from build123d import *

# Parameters (mm, degrees)
SKETCH1_R           = 2.65
BOSS_EXTRUDE1_DEPTH = 5
BOSS_EXTRUDE2_DEPTH = 10
SKETCH3_R           = 1.4
CUT_EXTRUDE1_DEPTH  = 16


with BuildPart() as part:
    # Sketch1 → Boss-Extrude1 (new body)
    with BuildSketch(Plane.XY):
        with BuildLine():
            Line((5, 28), (-5, 28))
            ThreePointArc((-5, 28), (-23.605754448, 19.060621125), (-28.253479924, -1.05119732))
            ThreePointArc((-28.253479924, -1.05119732), (-23.041182278, -4.770781049), (-18.77, 0))
            ThreePointArc((-18.77, 0), (0, 7.222918877), (18.77, 0))
            ThreePointArc((18.77, 0), (23.041182278, -4.770781049), (28.253479924, -1.05119732))
            ThreePointArc((28.253479924, -1.05119732), (23.605754448, 19.060621125), (5, 28))
        make_face()
        with Locations((-23.57, 0)):
            Circle(SKETCH1_R, mode=Mode.SUBTRACT)
        with Locations((23.57, 0)):
            Circle(SKETCH1_R, mode=Mode.SUBTRACT)
    extrude(amount=BOSS_EXTRUDE1_DEPTH)

    # Sketch2 → Boss-Extrude2 (add)
    with BuildSketch(Plane(origin=(0, 0, 0), x_dir=(-1, 0, 0), z_dir=(0, 0, -1))):
        with BuildLine():
            Line((-28.713948761, 6.537166667), (-6.158885262, 6.537166667))
            ThreePointArc((-6.158885262, 6.537166667), (0, 7.222918877), (6.158885262, 6.537166667))
            Line((6.158885262, 6.537166667), (28.713948761, 6.537166667))
            ThreePointArc((28.713948761, 6.537166667), (20.992221394, 21.837553063), (5, 28))
            Line((5, 28), (-5, 28))
            ThreePointArc((-5, 28), (-20.992221394, 21.837553063), (-28.713948761, 6.537166667))
        make_face()
    extrude(amount=BOSS_EXTRUDE2_DEPTH)

    # Sketch3 → Cut-Extrude1 (cut, through all)
    with BuildSketch(Plane(origin=(0, 0, -10), x_dir=(-1, 0, 0), z_dir=(0, 0, -1))):
        with Locations((0, 24.572918877)):
            Circle(SKETCH3_R)
        with Locations((0, 21.122918877)):
            Circle(SKETCH3_R)
        with Locations((0, 17.672918877)):
            Circle(SKETCH3_R)
        with Locations((0, 14.222918877)):
            Circle(SKETCH3_R)
    extrude(amount=-CUT_EXTRUDE1_DEPTH, mode=Mode.SUBTRACT)


solid = part.part
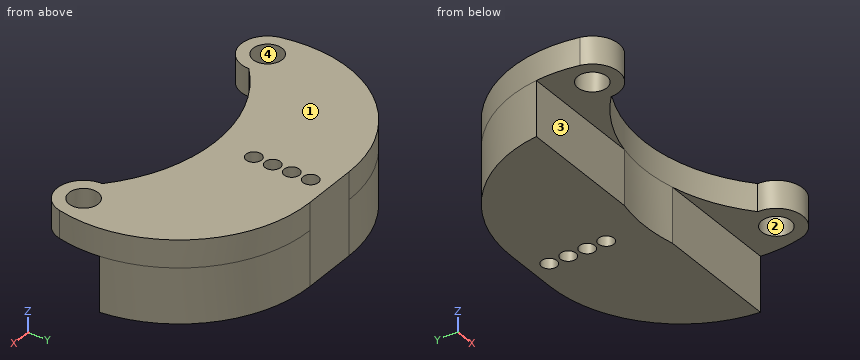
Input: part model. Units: mm. Frame: model coordinates. Face numbers are marked on the shaded views. A direction names the side the tool comes from. Coordinates: 2 decimals unless noted, no trailing zeros. Write each loop counter-clockwise with the first axis right and the second up, starting at its lowest first coordinate (ties: lowest second). Pieces come first, ordered by that corner, then holes. Notation, with made-up numbers: M 35.5,10.25 L 67.5,10.25 A32 cw 67.5,48.25 Z; hole C 2.25,4 d2. An arc over 180 degrees is marked long. Answer as a JSON object with one key per item and string values. Group by question number.
(1) Section A-A on x = 0. Output: boundary loops of the cut face in (y, z), plus the area to 3 significant figures.
(2) Section C-C on y = 1.5. Output: boundary loops of the cut face in (x, z).
(3) Section B-B on x = 23.57. Output: boundary loops of the cut face in (y, z), plus the area to 3 significant figures.
(4) Ray query, line 1 along Y through (x, z) = (0, -4.75); line 2 along X through (y, z) = (20.5, -7.5); line 3 along X through (y, z) = (-3, 3.25). Return the intervals inside material, ascending. Write a range as [from, to].
(5) Contact query for flat-ended pins moving along their axis: P1, Ø3.5, axis at x = 21, y = 2.5, coming from the -Z side; P2, Ø6, axis at y = 5, z = -3.5, coming from the +X side; P3, Ø12, axis at x = 2.5, y = 5, coming from the +Z side; P4, Ø1.5, axis at y = 16, z = -8, coming from the +X side. Output: stop coordinate, or through.
(6) Set-up query: the marked faces 3 and 4. Return all of +Z, -Z, +X, -X, +Y, -Y with unobstructed straight access to the full face (end or side cutting, diameter ignored); none if empty.
(7) Mould query, pull axis X, two halves, no side actions, for the marked faces 1 and 2. Classes: pulls with the +X half, pulls with the -X half, needs draft (parallel to the pull), parting line crosses it, or undercut.
(8) Section D-D on z = -4.75. Output: boundary loops of the cut face in (x, y).
Result set:
{
 "1": {"outline": "M 7.22,-10 L 12.82,-10 L 12.82,5 L 7.22,5 Z; M 15.62,-10 L 16.27,-10 L 16.27,5 L 15.62,5 Z; M 19.07,-10 L 19.72,-10 L 19.72,5 L 19.07,5 Z; M 22.52,-10 L 23.17,-10 L 23.17,5 L 22.52,5 Z; M 25.97,-10 L 28,-10 L 28,5 L 25.97,5 Z", "area": "144 mm2"},
 "2": {"outline": "M -28.68,0 L -25.75,0 L -25.75,5 L -28.68,5 Z; M -21.39,0 L -16.96,0 L -16.96,5 L -21.39,5 Z; M 16.96,0 L 21.39,0 L 21.39,5 L 16.96,5 Z; M 25.75,0 L 28.68,0 L 28.68,5 L 25.75,5 Z"},
 "3": {"outline": "M -4.8,0 L -2.65,0 L -2.65,5 L -4.8,5 Z; M 2.65,0 L 6.54,0 L 6.54,-10 L 19.11,-10 L 19.11,5 L 2.65,5 Z", "area": "219 mm2"},
 "4": {"line 1": "y = [7.22, 12.82], [15.62, 16.27], [19.07, 19.72], [22.52, 23.17], [25.97, 28]", "line 2": "x = [-22.36, -1.25], [1.25, 22.36]", "line 3": "x = [-27.32, -19.82], [19.82, 27.32]"},
 "5": {"P1": "stops at z = 0", "P2": "stops at x = 28.71", "P3": "stops at z = 5", "P4": "stops at x = 26.1"},
 "6": {"face 3": "-Z, +X, -X, -Y", "face 4": "+Z, -Z"},
 "7": {"face 1": "needs draft", "face 2": "undercut"},
 "8": {"outline": "M -28.71,6.54 L -6.16,6.54 A28 cw 6.16,6.54 L 28.71,6.54 A23.83 ccw 5,28 L -5,28 A23.83 ccw Z; hole C 0,14.22 d2.8; hole C 0,17.67 d2.8; hole C 0,21.12 d2.8; hole C 0,24.57 d2.8"}
}
